```python
from build123d import *

# Parameters (mm, degrees)
BOSS_EXTRUDE1_DEPTH = 5
SKETCH2_W           = 2
SKETCH2_H           = 3
CUT_EXTRUDE1_DEPTH  = 5
SKETCH3_W           = 2
SKETCH3_H           = 2.999556198
CUT_EXTRUDE2_DEPTH  = 15


with BuildPart() as part:
    # Sketch1 → Boss-Extrude1 (new body)
    with BuildSketch(Plane(origin=(0, 0, 0), x_dir=(1, 0, 0), z_dir=(0, 1, 0))):
        Polygon((0, 0), (6, 0), (6, 2), (5, 4), (4, 2), (2, 2), (1, 4), (0, 2), align=None)
    extrude(amount=BOSS_EXTRUDE1_DEPTH)

    # Sketch2 → Cut-Extrude1 (cut)
    with BuildSketch(Plane.XY):
        with Locations((3, 3.5)):
            Rectangle(SKETCH2_W, SKETCH2_H)
    extrude(amount=-CUT_EXTRUDE1_DEPTH, mode=Mode.SUBTRACT)

    # Sketch3 → Cut-Extrude2 (cut)
    with BuildSketch(Plane.ZY):
        with Locations((-1, 3.500221901)):
            Rectangle(SKETCH3_W, SKETCH3_H)
    extrude(amount=-CUT_EXTRUDE2_DEPTH, mode=Mode.SUBTRACT)


solid = part.part
```
Build history of the part. All positions in model axes, mm. A direction names the side the tool comes from. Coordinates: 2 decimals unless noted, no trailing zeros. Order: outer loops, then holes, each group sorted by start corner. A loop starts at its lowest first (then second) coordinate and runs counter-clockwise, first axis right, second up. Notation, with made-up numbers: M 70,-3 L 122,-3 A18 cw 122,9 Z; hole C -13,34.25 d6. An arc over 180 degrees is marked long. One line per question, with ' | ' between items. Start each with the question number.
1. Cut at A-A (y = 3.3). Write the cut outline in (x, z), plus the area to 3 significant figures.
2. Tool access for faces 1 (the face through (3, 1, -2)), 2 (the face through (1, 5, -3)), 3 (the face through (5, 3, -2)): list every direction of +Z, -Z, +X, -X, +Y, -Y with a clear straight run to the whole face (end or side of a thin tool).
3. Flat gauge pins, fed straight in: P1, Ø1.6, axis at x = 5, y = 4, coming from the +Z side; P2, Ø0.6, axis at x = 2.5, y = 1.5, coming from the -Z side; P3, Ø1.5, axis at x = 5, y = 1, coming from the -Z side. Where does each tip first touch, or does it go through?
4. Mould opens along X. For faces 4 (the face through (1.5, 2.5, -3)), 5 (the face through (6, 1, -1)), 6 (the face through (4.5, 2.5, -3)), 7 (the face through (5, 2, -1)) say: +X half, -X half, draft (parallel to the pull), parting line (faces both ways), or undercut.
5. Cut at C-C (x = 5.35). Write the cut outline in (y, z).
6. Cut at D-D (y = 1.05). Write the cut outline in (x, z).
7. Wall check: line 1 along Y through (x, z) = (5.05, -1.35); line 2 along X through (y, z) = (3.55, -2.6); line 3 along X through (y, z) = (2.25, -3.65) (3 decimals). Give the ranges that are in metal, low to high. Write a range as [from, to].
The answers:
1) outline: M 0,-2 L 1,-4 L 2,-2 Z; M 4,-2 L 5,-4 L 6,-2 Z | area: 4.00 mm2
2) face 1: -Z, +Y, -Y | face 2: +Z, -Z, +X, -X, +Y | face 3: +Z, +X, -X, +Y
3) P1: stops at z = -2 | P2: stops at z = -2 | P3: stops at z = -4
4) face 4: undercut | face 5: +X half | face 6: undercut | face 7: draft
5) outline: M 0,-3.3 L 5,-3.3 L 5,-2 L 2,-2 L 2,0 L 0,0 Z
6) outline: M 0,-2 L 1,-4 L 2,-2 L 4,-2 L 5,-4 L 6,-2 L 6,0 L 0,0 Z
7) line 1: y = [0, 2] | line 2: x = [0.3, 1.7], [4.3, 5.7] | line 3: x = [0.825, 1.175], [4.825, 5.175]
